Could you check a few things on this model? Use its own coordinates, in mm. A direction names the side the tool comes from. Give positions to 0.01 mm unless a question says otherwise; leave off trailing zeros. Loops run counter-clockwise (first coordinate to the right, second up) from the corner with the lowest first, then second, coordinate; pieces in that order, holes last. Notation, with made-up numbers: M 69.25,89.25 L 120.25,89.25 A18 cw 120.25,117.25 Z; hole C -23.5,-25 d5. An arc over 180 degrees is marked long. Use a Markdown table: item, result. Add a question column.
1) Suppose I cut it at D-D on z = 3. List the corners of the cut face in (x, y) for me, and give its area (3 significant figures).
2) We'd pull the mould along Z, two halves only. Please class faces 4 (the flat face through (-20, 4, -26.5)), 5 (the flat face through (-14, 33, 47.5)), 6 (the flat face through (-13, 21, -47.5)), 7 (the flat face through (-0.67, 44.49, 45.04)): +Z half, -Z half, draft (parallel to the pull), parting line (faces both ways), or undercut.
3) Suppose I cut it at A-A on z = 15. List the corners of the cut face in (x, y) for me, and give its area (4 significant figures).
4) Suppose I cut it at C-C on y = 32. List the corners of the cut face in (x, z) for me, and give its area (3 significant figures).
5) Will these pins go through, and if not, where does the flat tip stop? pin 1 Ø2 at (x, z) = (-5.5, -2.5) entering from -Y; pin 2 Ø4 at (x, y) = (33, 28) entering from +Z.
6) Suppose I cut it at B-B on x = -63.5. List the corners of the cut face in (y, z) for me, and give its area (3 significant figures).
7) Which directions (+Z, -Z, +X, -X, +Y, -Y) give clear straight access to the entire face, cutting with the end or side of a thin tool? Please do faces 1 (the flat face through (-36, 3, 20)), 2 (the flat face through (-15, 4, 29.5)), 3 (the flat face through (-53, 76, 37.5)).
8) If I drill on line 1 along X through (y, z) = (3.4, 3); line 2 along Z through (x, y) = (-36.5, 40); line 3 along Z through (x, y) = (-63.5, 3), over which ranges is the centre line in solid material (lowest first)? Write a range as [from, to].
```python
from build123d import *

# Parameters (mm, degrees)
SKETCH1_W           = 132
SKETCH1_H           = 95
BOSS_EXTRUDE1_DEPTH = 6
SKETCH3_W           = 10
SKETCH3_H           = 20
CUT_EXTRUDE2_DEPTH  = 10
CUT_EXTRUDE3_DEPTH  = 5
BOSS_EXTRUDE2_DEPTH = 4.5
BOSS_EXTRUDE3_DEPTH = 5
SKETCH9_R           = 1.75
CUT_EXTRUDE4_DEPTH  = 10
SKETCH10_W          = 13
SKETCH10_H          = 10
BOSS_EXTRUDE4_DEPTH = 2.5
SKETCH12_R          = 1.75
CUT_EXTRUDE6_DEPTH  = 4


with BuildPart() as part:
    # Sketch1 → Boss-Extrude1 (new body)
    with BuildSketch(Plane(origin=(0, 0, 0), x_dir=(1, 0, 0), z_dir=(0, 1, 0))):
        Rectangle(SKETCH1_W, SKETCH1_H)
    extrude(amount=BOSS_EXTRUDE1_DEPTH)

    # Sketch3 → Cut-Extrude2 (cut)
    with BuildSketch(Plane(origin=(0, 6, 0), x_dir=(1, 0, 0), z_dir=(0, 1, 0))):
        with Locations((-31, -19.5)):
            Rectangle(SKETCH3_W, SKETCH3_H)
    extrude(amount=-CUT_EXTRUDE2_DEPTH, mode=Mode.SUBTRACT)

    # Sketch4 → Cut-Extrude3 (cut)
    with BuildSketch(Plane(origin=(0, 6, 0), x_dir=(1, 0, 0), z_dir=(0, 1, 0))):
        Polygon((-11.15, 24), (-11.15, 11.5), (-19, 11.5), (-19, -29.5), (-11.15, -29.5), (-11.15, -39), (-8.65, -39), (33.2, -39), (35.7, -39), (35.7, -29), (41.7, -29), (41.7, 33), (35.7, 33), (35.7, 40.5), (66, 40.5), (66, 43), (35.7, 43), (33.2, 43), (33.2, 33), (27.2, 33), (27.2, -29), (33.2, -29), (33.2, -36.5), (-8.65, -36.5), (-8.65, -29.5), (-0.8, -29.5), (-0.8, 11.5), (-8.65, 11.5), (-8.65, 26.5), (-11.15, 26.5), (-32.25, 26.5), (-32.25, 24), (-32.25, -9.5), (-29.75, -9.5), (-29.75, 24), align=None)
    extrude(amount=-CUT_EXTRUDE3_DEPTH, mode=Mode.SUBTRACT)

    # Sketch6 → Boss-Extrude2 (add)
    with BuildSketch(Plane(origin=(0, 0, -47.5), x_dir=(-1, 0, 0), z_dir=(0, 0, -1))):
        Polygon((66, 6), (66, 82.210235533), (-66, 6), align=None)
    extrude(amount=-BOSS_EXTRUDE2_DEPTH)

    # Sketch7 → Boss-Extrude3 (add)
    with BuildSketch(Plane.XY.offset(47.5)):
        Polygon((-66, 6), (-66, 82.210235533), (66, 6), align=None)
    extrude(amount=-BOSS_EXTRUDE3_DEPTH)

    # Sketch9 → Cut-Extrude4 (cut)
    with BuildSketch(Plane.XZ):
        with Locations(Location((63.5, 3, 0), (0, 0, 270))):
            Circle(SKETCH9_R)
        with Locations(Location((-63.5, 3, 0), (0, 0, 90))):
            Circle(SKETCH9_R)
    extrude(amount=-CUT_EXTRUDE4_DEPTH, mode=Mode.SUBTRACT)

    # Sketch10 → Boss-Extrude4 (add)
    with BuildSketch(Plane(origin=(19.098076211, 33.078838325, 0), x_dir=(0.8660254037844417, -0.49999999999999495, 0), z_dir=(0.49999999999999495, 0.8660254037844417, 0))):
        with Locations((-83.552558883, 42.5)):
            Rectangle(SKETCH10_W, SKETCH10_H)
        with Locations((39.447441117, 42.5)):
            Rectangle(SKETCH10_W, SKETCH10_H)
        with Locations((-83.552558883, -42.5)):
            Rectangle(SKETCH10_W, SKETCH10_H)
        with Locations((39.447441117, -42.5)):
            Rectangle(SKETCH10_W, SKETCH10_H)
    extrude(amount=BOSS_EXTRUDE4_DEPTH)

    # Sketch12 → Cut-Extrude6 (cut)
    with BuildSketch(Plane(origin=(20.348076211, 35.243901834, 0), x_dir=(0.8660254037844417, -0.4999999999999949, 0), z_dir=(0.4999999999999949, 0.8660254037844417, 0))):
        with Locations(Location((39.447441117, 42.5, 0), (0, 0, 180))):
            Circle(SKETCH12_R)
        with Locations(Location((-83.552558883, 42.5, 0), (0, 0, 180))):
            Circle(SKETCH12_R)
        with Locations(Location((-83.552558883, -42.5, 0), (0, 0, 180))):
            Circle(SKETCH12_R)
        with Locations(Location((39.447441117, -42.5, 0), (0, 0, 180))):
            Circle(SKETCH12_R)
    extrude(amount=-CUT_EXTRUDE6_DEPTH, mode=Mode.SUBTRACT)


solid = part.part
```
Answer block:
| question | item | result |
|---|---|---|
| 1 | outline | M -66,0 L -65.25,0 L -65.25,6 L -66,6 Z; M -61.75,0 L 61.75,0 L 61.75,6 L 41.7,6 L 41.7,1 L 27.2,1 L 27.2,6 L -0.8,6 L -0.8,1 L -19,1 L -19,6 L -29.75,6 L -29.75,1 L -32.25,1 L -32.25,6 L -61.75,6 Z; M 65.25,0 L 66,0 L 66,6 L 65.25,6 Z |
| 1 | area | 574 mm^2 |
| 2 | face 4 | undercut |
| 2 | face 5 | +Z half |
| 2 | face 6 | -Z half |
| 2 | face 7 | draft |
| 3 | outline | M -66,0 L -36,0 L -36,6 L -66,6 Z; M -26,0 L 66,0 L 66,6 L 41.7,6 L 41.7,1 L 27.2,1 L 27.2,6 L -0.8,6 L -0.8,1 L -19,1 L -19,6 L -26,6 Z |
| 3 | area | 568.5 mm^2 |
| 4 | outline | M -66,-47.5 L 20.97,-47.5 L 20.97,-43 L -66,-43 Z; M -66,42.5 L 20.97,42.5 L 20.97,47.5 L -66,47.5 Z |
| 4 | area | 826 mm^2 |
| 5 | pin 1 | stops at y = 0 |
| 5 | pin 2 | passes through |
| 6 | outline | M 0,-47.5 L 80.77,-47.5 L 80.77,-43 L 6,-43 L 6,1.25 L 0,1.25 Z; M 0,4.75 L 6,4.75 L 6,42.5 L 80.77,42.5 L 80.77,47.5 L 0,47.5 Z |
| 6 | area | 1,260 mm^2 |
| 7 | face 1 | +Y, -Y |
| 7 | face 2 | +Y |
| 7 | face 3 | +X, -X, +Y |
| 8 | line 1 | x = [-66, -65.25], [-61.75, -32.25], [-29.75, -19], [-0.8, 27.2], [41.7, 61.75], [65.25, 66] |
| 8 | line 2 | z = [-47.5, -43], [42.5, 47.5] |
| 8 | line 3 | z = [-47.5, 1.25], [4.75, 47.5] |
